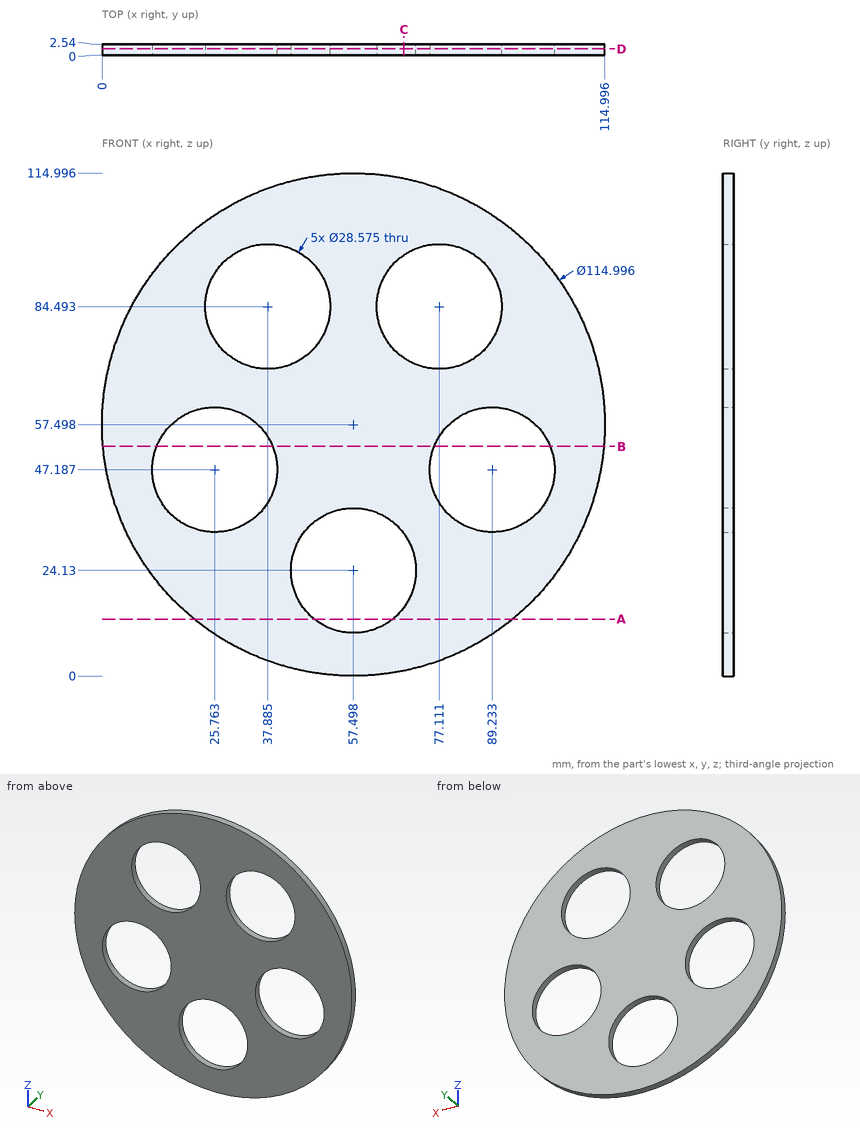
For this review, use the dimensioned drawing (mm, ordinates from the lowest corner) and the shaded views. Give positions to 0.01 mm unless a question says otherwise; leave off trailing zeros. Loops run counter-clockwise (first coordinate to the right, second up) from the corner with the lowest first, then second, coordinate; pieces in that order, holes last.
Item 1: Insertion check: pin 1 (2 mm diameter, centred on x = 71, z = 60.5, fed in from -Y); pin 2 (1.5 mm diameter, centred on y = 1, z = 82.5, fed in from -X) (1 decimal). Each pin has a flat end and moves straight along its axis. Give the tip position at first contact, or say it passes through.
Item 2: For line 1 along Z through (x, y) = (86, 1.85) (1 decimal); line 2 along X through (y, z) = (1.95, 88) (1 decimal); line 3 along X through (y, z) = (0.8, 48.5) (1 decimal), list the stretches that pass through material, from the lowest coordinate up.
Item 3: Take a section at D-D, the plane y = 1.4. State the section outline as (x, z) points (1 decimal), and give its area (3 significant figures).
Item 4: Take a section at B-B, the plane z = 52.5. State the section outline as (x, y) points (1 decimal), and give its area (3 significant figures).
Item 5: Take a section at A-A, the plane z = 13. State the section outline as (x, y) points (1 decimal).
Item 6: Take a section at C-C, the plane x = 69. State the section outline as (y, z) points (1 decimal).
Calculated:
1. pin 1: stops at y = 0
1. pin 2: stops at x = 5.4
2. line 1: z = 7.6 to 33.3, 61.1 to 73.3, 95.7 to 107.4
2. line 2: x = 8.8 to 24, 51.7 to 63.3, 91 to 106.2
2. line 3: x = 0.7 to 11.5, 40 to 75, 103.5 to 114.3
3. outline: circle Ø115 at (57.5, 57.5); hole circle Ø28.6 at (25.8, 47.2); hole circle Ø28.6 at (37.9, 84.5); hole circle Ø28.6 at (57.5, 24.1); hole circle Ø28.6 at (77.1, 84.5); hole circle Ø28.6 at (89.2, 47.2)
3. area: 7,180 mm2
4. outline: (0.2, 0) - (12.5, 0) - (12.5, 2.5) - (0.2, 2.5) - close; (39, 0) - (76, 0) - (76, 2.5) - (39, 2.5) - close; (102.5, 0) - (114.8, 0) - (114.8, 2.5) - (102.5, 2.5) - close
4. area: 156 mm2
5. outline: (21.1, 0) - (48.5, 0) - (48.5, 2.5) - (21.1, 2.5) - close; (66.5, 0) - (93.9, 0) - (93.9, 2.5) - (66.5, 2.5) - close
6. outline: (0, 1.2) - (2.5, 1.2) - (2.5, 15.7) - (0, 15.7) - close; (0, 32.6) - (2.5, 32.6) - (2.5, 72.7) - (0, 72.7) - close; (0, 96.3) - (2.5, 96.3) - (2.5, 113.8) - (0, 113.8) - close
